```python
from build123d import *

# Parameters (mm, degrees)
PAD_DEPTH    = 10
PAD001_DEPTH = 10
SKETCH002_R  = 1.5
POCKET_DEPTH = 10.001


with BuildPart() as part:
    # Sketch → Pad (new body)
    with BuildSketch(Plane.XY):
        with BuildLine():
            ThreePointArc((25.669873, 10), (26.447689, 5.961126), (28.669873, 2.5))
            Line((28.669873, 2.5), (42.669873, 2.5))
            ThreePointArc((42.669873, 2.5), (44.892057, 5.961126), (45.669873, 10))
            Line((48.169873, 10), (45.669873, 10))
            Line((48.169873, 0), (48.169873, 10))
            Line((23.169873, 0), (48.169873, 0))
            Line((23.169873, 0), (23.169873, 7.5))
            Line((23.169873, 7.5), (0, 7.5))
            ThreePointArc((0, 7.5), (-1.25, 7.165064), (-2.165064, 6.25))
            ThreePointArc((-4.330127, 10), (-6.495191, 6.25), (-2.165064, 6.25))
            Line((-4.330127, 10), (23.169873, 10))
            Line((25.669873, 10), (23.169873, 10))
        make_face()
    extrude(amount=PAD_DEPTH)

    # Sketch001 (on Face12 of Pad) → Pad001 (join)
    with BuildSketch(Plane.XY.offset(10)):
        Polygon((48.169873, 10), (48.169873, 8), (50.169873, 8), (50.169873, 6), (52.169873, 6), (52.169873, 10), align=None)
    extrude(amount=-PAD001_DEPTH)

    # Sketch002 (on Face17 of Pad001) → Pocket (cut, through all)
    with BuildSketch(Plane.XY.offset(10)):
        with Locations((-4.330127, 7.5)):
            Circle(SKETCH002_R)
    extrude(amount=-POCKET_DEPTH, mode=Mode.SUBTRACT)


solid = part.part
```
Source: CAD feature listing. Evaluate the final solid. Frame: model axes, mm. A direction names the side the tool comes from. Give positions to 0.01 mm unless a question says otherwise; leave off trailing zeros. Loops run counter-clockwise (first coordinate to the right, second up) from the corner with the lowest first, then second, coordinate; pieces in that order, holes last. Notation, with made-up numbers: (53.25, -33.75) - (70.25, -33.75) arc R30 cw to (70.25, 2.25) - close; hole circle Ø6 at (60, 22). An arc over 180 degrees is marked (long way). Use CSV: the item, a comma, the result in double quotes. Start each with the question number.
1. Pin query (flat end, axial travel): pin 1 (1 mm diameter, centred on x = 17.5, z = 6.5, fed in from -Y); pin 2 (3 mm diameter, centred on x = 38.5, z = 1, fed in from -Y); pin 3 (1.6 mm diameter, centred on x = 49.5, z = 3, fed in from -Y); pin 4 (1.5 mm diameter, centred on y = 1.5, z = 7.5, fed in from -X). Return the tip coordinate at first contact, or that it passes through.
2. Draft query along X for faces 1 (the flat face through (48.17, 4, 5)), 2 (the flat face through (52.17, 8, 5)), 3 (the cylindrical face through (44.87, 5.91, 4.93)), 4 (the flat face through (25, 5, 0)). Return one class per face: +X half, -X half, draft (parallel to the pull), parting line (faces both ways), or undercut.
3. Section A-A (z = 3). Output: boundary loops of the cut face in (x, y) (3 decimals), then the cut area to 3 significant figures.
4. Section C-C (x = 10.5). Output: boundary loops of the cut face in (y, z).
5. Ray query, L1, parallel to X at y = 5.5, z = 0.5; L2, parallel to X at y = 6.5, z = 1.5; L3, parallel to X at y = 7.75, z = 3. Return the intervals inside material, ascending.
6. Reachability of faces 5 (the flat face through (12, 7.5, 5)), 6 (the flat face through (25, 5, 10)), 7 (the cylindrical face through (26.43, 6.01, 4.93)), 8 (the flat face through (51, 6, 5)) from +Z, -Z, +X, -X, +Y, -Y: full face, straight path, thin tool, end or side. Return the list, or none.
7. Section D-D (y = 1). Output: boundary loops of the cut face in (x, z), then the cut area to 3 significant figures.
8. Section B-B (y = 4.5). Output: boundary loops of the cut face in (x, z).
Response:
1,pin 1,"y = 7.5"
1,pin 2,"y = 0"
1,pin 3,"y = 6"
1,pin 4,"x = 23.17"
2,face 1,"undercut"
2,face 2,"+X half"
2,face 3,"undercut"
2,face 4,"draft"
3,outline,"(-4.33, 10) arc R2.5 ccw (long way) to (-2.165, 6.25) arc R2.5 cw to (0, 7.5) - (23.17, 7.5) - (23.17, 0) - (48.17, 0) - (48.17, 8) - (50.17, 8) - (50.17, 6) - (52.17, 6) - (52.17, 10) - (45.67, 10) arc R10.875 cw to (42.67, 2.5) - (28.67, 2.5) arc R10.875 cw to (25.67, 10) - close; hole circle Ø3 at (-4.33, 7.5)"
3,area,"203 mm²"
4,outline,"(7.5, 0) - (10, 0) - (10, 10) - (7.5, 10) - close"
5,L1,"-5.83 to -2.83, 23.17 to 26.64, 44.7 to 48.17"
5,L2,"-6.62 to -5.45, -3.21 to -2, 23.17 to 26.25, 45.09 to 48.17, 50.17 to 52.17"
5,L3,"-6.82 to -5.81, -2.85 to 25.91, 45.43 to 48.17, 50.17 to 52.17"
6,face 5,"+Z, -Z, -Y"
6,face 6,"+Z, +X, -X, +Y, -Y"
6,face 7,"+Z, -Z, +Y"
6,face 8,"+Z, -Z, +X, -Y"
7,outline,"(23.17, 0) - (48.17, 0) - (48.17, 10) - (23.17, 10) - close"
7,area,"250 mm²"
8,outline,"(23.17, 0) - (27.16, 0) - (27.16, 10) - (23.17, 10) - close; (44.18, 0) - (48.17, 0) - (48.17, 10) - (44.18, 10) - close"
